```python
from build123d import *

# Parameters (mm, degrees)
BOSS_EXTRU_1_DEPTH      = 2
ESQUISSE4_R             = 1.5
ENL_V_MAT_EXTRU_1_DEPTH = 10


with BuildPart() as part:
    # Esquisse1 → Boss.-Extru.1 (new body)
    with BuildSketch(Plane(origin=(0, 0, 0), x_dir=(1, 0, 0), z_dir=(0, 1, 0))):
        with BuildLine():
            Line((-51.25, 0), (-51.25, -34.62957381))
            Line((-51.25, -34.62957381), (-43.25, -34.62957381))
            Line((-43.25, -34.62957381), (-43.25, -46.62957381))
            Line((-43.25, -46.62957381), (-51.25, -46.62957381))
            Line((-51.25, -46.62957381), (-51.25, -88.75))
            Line((-51.25, -88.75), (51.25, -88.75))
            Line((51.25, -88.75), (51.25, 0))
            ThreePointArc((51.25, 0), (0, 51.25), (-51.25, 0))
        make_face()
    extrude(amount=BOSS_EXTRU_1_DEPTH)

    # Esquisse4 → Enlèv. mat.-Extru.1 (cut)
    with BuildSketch(Plane(origin=(0, 2, 0), x_dir=(1, 0, 0), z_dir=(0, 1, 0))):
        with Locations(Location((15, 30, 0), (0, 0, 270))):
            Circle(ESQUISSE4_R)
        with Locations(Location((-15, 30, 0), (0, 0, 270))):
            Circle(ESQUISSE4_R)
    extrude(amount=-ENL_V_MAT_EXTRU_1_DEPTH, mode=Mode.SUBTRACT)


solid = part.part
```
Model file for the job. Use its own axes, mm. Coordinates: 2 decimals unless noted, no trailing zeros. Order: outer loops, then holes, each group sorted by start corner. A loop starts at its lowest first (then second) coordinate and runs counter-clockwise, first axis right, second up. Notation, with made-up numbers: (-19, -18) - (-5, -18) arc R20 cw to (-5, -12) - close; hole circle Ø10 at (-1, 10). An arc over 180 degrees is marked (long way). Return JSON: item names as keys, results as strings. Group by question number.
1) Saw through at A-A, the plane y = 1.6. Write the cut outline in (x, z), plus the area to 3 significant figures.
2) Probe line 1 (X direction, y = 1, z = -30); line 2 (X direction, y = 0.25, z = 38); line 3 (Z direction, x = -14, y = 0.3). List the from-to ranges inside material, lowest first. Write a range as from..to.
3) Mould opens along X. For faces 1 (the flat face through (-1, 0, 18)), 2 (the cylindrical face through (-14.93, 1.01, -31.5)), 3 (the cylindrical face through (1.127, 0.986, -51.238)) say: released by +X, released by -X, zero draft, split by the parting line, or undercut.
4) Saw through at D-D, the plane x = -31. Write the cut outline in (y, z), plus the area to 3 significant figures.
5) Flat gauge pin, fed straight in: P1, Ø2, axis at x = -24, z = -30, coming from the -Y side. Where does the tip first touch, or does it go through?
6) Saw through at C-C, the plane z = -30. Write the cut outline in (x, y), plus the area to 3 significant figures.
7) Saw through at B-B, the plane x = 15. Write the cut outline in (y, z).
Values found:
{
 "1": {"outline": "(-51.25, 0) arc R51.25 ccw to (51.25, 0) - (51.25, 88.75) - (-51.25, 88.75) - (-51.25, 46.63) - (-43.25, 46.63) - (-43.25, 34.63) - (-51.25, 34.63) - close; hole circle Ø3 at (-15, -30); hole circle Ø3 at (15, -30)", "area": "13,100 mm²"},
 "2": {"line 1": "x = -41.55..-16.5, -13.5..13.5, 16.5..41.55", "line 2": "x = -43.25..51.25", "line 3": "z = -49.3..-31.12, -28.88..88.75"},
 "3": {"face 1": "zero draft", "face 2": "undercut", "face 3": "split by the parting line"},
 "4": {"outline": "(0, -40.81) - (2, -40.81) - (2, 88.75) - (0, 88.75) - close", "area": "259 mm²"},
 "5": {"P1": "stops at y = 0"},
 "6": {"outline": "(-41.55, 0) - (-16.5, 0) - (-16.5, 2) - (-41.55, 2) - close; (-13.5, 0) - (13.5, 0) - (13.5, 2) - (-13.5, 2) - close; (16.5, 0) - (41.55, 0) - (41.55, 2) - (16.5, 2) - close", "area": "154 mm²"},
 "7": {"outline": "(0, -49.01) - (2, -49.01) - (2, -31.5) - (0, -31.5) - close; (0, -28.5) - (2, -28.5) - (2, 88.75) - (0, 88.75) - close"}
}
